```python
from build123d import *

# Parameters (mm, degrees)
SKETCH_1_R          = 18.5
EXTRUDE_1_DEPTH     = 23
SKETCH_3_R          = 16.5
EXTRUDE_2_DEPTH     = 22.5
SKETCH_4_R          = 1.5
CUT_EXTRUDE_1_DEPTH = 15
SKETCH_5_R          = 6
EXTRUDE_3_DEPTH     = 6
SKETCH_6_R          = 3
EXTRUDE_4_DEPTH     = 12


with BuildPart() as part:
    # 草图1 → 凸台-拉伸1 (new body)
    with BuildSketch(Plane(origin=(0, 0, 0), x_dir=(1, 0, 0), z_dir=(0, 1, 0))):
        with Locations(Location((0, 0, 0), (0, 0, 270))):
            Circle(SKETCH_1_R)
    extrude(amount=-EXTRUDE_1_DEPTH)

    # 草图3 → 凸台-拉伸2 (add)
    with BuildSketch(Plane.XZ.offset(23)):
        with Locations(Location((0, 0, 0), (0, 0, 90))):
            Circle(SKETCH_3_R)
    extrude(amount=EXTRUDE_2_DEPTH)

    # 草图4 → 切除-拉伸1 (cut)
    with BuildSketch(Plane(origin=(0, 0, 0), x_dir=(1, 0, 0), z_dir=(0, 1, 0))):
        with Locations(Location((0, 15.5, 0), (0, 0, 270))):
            Circle(SKETCH_4_R)
        with Locations(Location((13.423393759, 7.75, 0), (0, 0, 270))):
            Circle(SKETCH_4_R)
        with Locations(Location((13.423393759, -7.75, 0), (0, 0, 270))):
            Circle(SKETCH_4_R)
        with Locations(Location((0, -15.5, 0), (0, 0, 270))):
            Circle(SKETCH_4_R)
        with Locations(Location((-13.423393759, -7.75, 0), (0, 0, 270))):
            Circle(SKETCH_4_R)
        with Locations(Location((-13.423393759, 7.75, 0), (0, 0, 270))):
            Circle(SKETCH_4_R)
    extrude(amount=-CUT_EXTRUDE_1_DEPTH, mode=Mode.SUBTRACT)

    # 草图5 → 凸台-拉伸3 (add)
    with BuildSketch(Plane(origin=(0, 0, 0), x_dir=(1, 0, 0), z_dir=(0, 1, 0))):
        with Locations(Location((0, 7, 0), (0, 0, 270))):
            Circle(SKETCH_5_R)
    extrude(amount=EXTRUDE_3_DEPTH)

    # 草图6 → 凸台-拉伸4 (add)
    with BuildSketch(Plane(origin=(0, 6, 0), x_dir=(1, 0, 0), z_dir=(0, 1, 0))):
        with Locations(Location((0, 7, 0), (0, 0, 270))):
            Circle(SKETCH_6_R)
    extrude(amount=EXTRUDE_4_DEPTH)


solid = part.part
```
CAD build for the part. Positions are in the model's coordinates, mm. A direction names the side the tool comes from. Round coordinates to 2 decimals unless told otherwise and drop trailing zeros. Order: outer loops, then holes, each group sorted by start corner. A loop starts at its lowest first (then second) coordinate and runs counter-clockwise, first axis right, second up.
Item 1: Saw through at B-B on z = 0. Write the cut outline in (x, y).
Item 2: Saw through at C-C on y = 7. Write the cut outline in (x, z).
Item 3: Probe line 1 along X through (y, z) = (-9.25, 7.75); line 2 along Y through (x, z) = (-15.5, 1); line 3 along Y through (x, z) = (-11, 12.5). List the from-to ranges inside material, lowest first.
Item 4: Mould opens along X. For faces 1 (the face through (16.108, -34.092, -3.577)), 2 (the face through (0, -7, -17)), 3 (the face through (0, 0, 0)) say: pulls with the +X half, pulls with the -X half, needs draft (parallel to the pull), parting line crosses it, or undercut.
Item 5: Tool access for faces 4 (the face through (-7.086, -11.339, 17.089)), 5 (the face through (-13, -15, 8)), 6 (the face through (0, -23, -17)): list every direction of +Z, -Z, +X, -X, +Y, -Y with a clear straight run to the whole face (end or side of a thin tool).
Item 6: Saw through at A-A on x = 0. Write the cut outline in (y, z), then the cut area to 3 significant figures.
Item 7: Pin check, flat tips, straight feed: pin 1 (4 mm diameter, centred on x = 13.42, z = -7.75, fed in from +Y); pin 2 (0.9 mm diameter, centred on x = -0.5, z = 16, fed in from +Y); pin 3 (3 mm diameter, centred on y = -30.5, z = 11, fed in from -X). Stop position of each tip, or through.
Item 8: Saw through at D-D on y = -14. Write the cut outline in (x, z).
Reported:
1. outline: (-18.5, -23) - (-16.5, -23) - (-16.5, -45.5) - (16.5, -45.5) - (16.5, -23) - (18.5, -23) - (18.5, 0) - (-18.5, 0) - close
2. outline: circle Ø6 at (0, -7)
3. line 1: x = -16.8 to -14.92, -11.92 to 11.92, 14.92 to 16.8
3. line 2: y = -45.5 to 0
3. line 3: y = -23 to 0
4. face 1: parting line crosses it
4. face 2: undercut
4. face 3: needs draft
5. face 4: +Y, -Y
5. face 5: +Y
5. face 6: -Y
6. outline: (-45.5, -16.5) - (-23, -16.5) - (-23, -18.5) - (0, -18.5) - (0, -17) - (-15, -17) - (-15, -14) - (0, -14) - (0, -13) - (6, -13) - (6, -10) - (18, -10) - (18, -4) - (6, -4) - (6, -1) - (0, -1) - (0, 14) - (-15, 14) - (-15, 17) - (0, 17) - (0, 18.5) - (-23, 18.5) - (-23, 16.5) - (-45.5, 16.5) - close
6. area: 1,650 mm2
7. pin 1: stops at y = 0
7. pin 2: stops at y = -15
7. pin 3: stops at x = -13.49
8. outline: circle Ø37 at (0, 0); hole circle Ø3 at (-13.42, -7.75); hole circle Ø3 at (-13.42, 7.75); hole circle Ø3 at (0, -15.5); hole circle Ø3 at (0, 15.5); hole circle Ø3 at (13.42, -7.75); hole circle Ø3 at (13.42, 7.75)
